Design review of the part built by this model. Coordinates are the model's own, in mm. A direction names the side the tool comes from. Round coordinates to 2 decimals unless told otherwise and drop trailing zeros. Order: outer loops, then holes, each group sorted by start corner. A loop starts at its lowest first (then second) coordinate and runs counter-clockwise, first axis right, second up. Notation, with made-up numbers: M -38,-19.75 L 7,-19.75 A17 cw 7,-3.75 Z; hole C -26.75,25.5 d5. An arc over 180 degrees is marked long. Use a Markdown table: item, result. Add a question column.
(1) Take a section at D-D (x = 10.5). Write out the cut boundary in (y, z) (3 decimals).
(2) For pin 1 (9.5 mm diameter, centred on x = 1.5, z = 4.5, fed in from -Y); pin 2 (1 mm diameter, centred on y = 2.5, z = 2, fed in from -X); pin 3 (1.5 mm diameter, centred on x = 8.5, y = 5.5, fed in from +Z), all flat-tipped, find the tip position at first contact; note any pin that passes through.
(3) Take a section at A-A (x = 0). Count the separate pieces of the cut face and the enclosed holes in it, then the cut area to 3 significant figures.
(4) The part is to be moulded in two halves that separate along X. For faces 3 (the face through (11, 0, 12)), 4 (the face through (0.06, 3.13, 26.1)), 5 (the face through (-15.2, 1.6, -4.8)), say which applies: released by +X, released by -X, zero draft, split by the parting line, or undercut.
(5) Machinability: for faces 1 (the face through (11, 3.175, -7)), 2 (the face through (-1.006, 3.219, 17.823)), which of the approach directions +Z, -Z, +X, -X, +Y, -Y give a long, thin tool a straight path to every point of the face, cutting with its end or side? Answer none if there is none.
(6) To check wall thickness, follow probe 1 along Z at (x, y) = (0, 2.5); probe 2 along Z at (x, y) = (0, 3.25); probe 3 along Y at (x, z) = (3, 13.5) (3 decimals). State the ranges of each line that lie inside material, in increasing order. Write a range as from..to.
Autodesk Inventor part; units mm, degrees
ref_plane "YZ Plane" through (0, 0, 0) normal (1, 0, 0) x (0, 1, 0)
ref_plane "XZ Plane" through (0, 0, 0) normal (0, 1, 0) x (-1, 0, 0)
ref_plane "XY Plane" through (0, 0, 0) normal (0, 0, 1) x (1, 0, 0)
sketch "Sketch1" plane through (0, 0, 0) normal (0, 1, 0) x (-1, 0, 0)
  circle A0 centre (0, 0) radius 12.7
  circle A1 centre (0, 0) radius 18.0975
  circle A2 centre (0, 21.0185) radius 5.08 construction
  circle A3 centre (0, -21.0185) radius 5.08 construction
  line L0 (3.9884, 24.1647) -> (14.2088, 11.2084)
  line L1 (-3.9884, 24.1647) -> (-14.2088, 11.2084)
  line L2 (-14.2088, -11.2084) -> (-3.9884, -24.1647)
  line L3 (3.9884, -24.1647) -> (14.2088, -11.2084)
  arc A4 (14.2088, -11.2084) -> (14.2088, 11.2084) centre (0, 0) ccw
  arc A5 (-3.9884, -24.1647) -> (3.9884, -24.1647) centre (0, -21.0185) ccw
  arc A6 (-14.2088, 11.2084) -> (-14.2088, -11.2084) centre (0, 0) ccw
  arc A7 (3.9884, 24.1647) -> (-3.9884, 24.1647) centre (0, 21.0185) ccw
  circle A8 centre (0, 0) radius 15.9385
  dimension "d0" = 25.4
  dimension "d1" = 36.195
  dimension "d2" = 10.16
  dimension "d7" = 31.877
  dimension "d15" = 42.037
extrude "Extrusion1" add sketch "Sketch1" along normal blind 6.35 contours A1 | A1 L1 A7 L0 | L3 A5 L2 A1 | A8
extrude "Extrusion2" cut sketch "Sketch1" along normal blind 3.175 contours A8
hole "Hole1" at (0, 0, 21.0185) at (0, 0, -21.0185) direction (0, 1, 0) diameter 6.7 end through all
properties part number "Retainer" material "ABS Plastic"
Verdict:
| question | item | result |
|---|---|---|
| 1 | outline | M 0,-15.91 L 6.35,-15.91 L 6.35,-7.144 L 3.175,-7.144 L 3.175,-11.991 L 0,-11.991 Z; M 0,11.991 L 3.175,11.991 L 3.175,7.144 L 6.35,7.144 L 6.35,15.91 L 0,15.91 Z |
| 2 | pin 1 | passes through |
| 2 | pin 2 | stops at x = -18.04 |
| 2 | pin 3 | stops at z = 19.4 |
| 3 | separate pieces | 4 |
| 3 | enclosed holes | 0 |
| 3 | area | 64.5 mm^2 |
| 4 | face 3 | zero draft |
| 4 | face 4 | split by the parting line |
| 4 | face 5 | undercut |
| 5 | face 1 | -Y |
| 5 | face 2 | +Y, -Y |
| 6 | probe 1 | z = -26.1..-24.37, -17.67..-15.94, 15.94..17.67, 24.37..26.1 |
| 6 | probe 2 | z = -26.1..-24.37, -17.67..-12.7, 12.7..17.67, 24.37..26.1 |
| 6 | probe 3 | y = 3.175..6.35 |
